from build123d import *

# Parameters (mm, degrees)
SKETCH_R        = 5
SKETCH_R_2      = 3.2
PAD_DEPTH       = 15
SKETCH002_R     = 6.1
POCKET001_DEPTH = 4
SKETCH003_R     = 11.1
POCKET_DEPTH    = 7.4


with BuildPart() as part:
    # Sketch → Pad (new body)
    with BuildSketch(Plane.XY):
        Polygon((20, 30), (20, 58), (62.3, 58), (62.3, 30), (82.3, 30), (82.3, 0), (0, 0), (0, 30), align=None)
        with Locations((41.15, 36.85)):
            Circle(SKETCH_R, mode=Mode.SUBTRACT)
        with Locations((11.15, 10)):
            Circle(SKETCH_R_2, mode=Mode.SUBTRACT)
        with Locations((31.15, 10)):
            Circle(SKETCH_R_2, mode=Mode.SUBTRACT)
        with Locations((51.15, 10)):
            Circle(SKETCH_R_2, mode=Mode.SUBTRACT)
        with Locations((71.15, 10)):
            Circle(SKETCH_R_2, mode=Mode.SUBTRACT)
    extrude(amount=PAD_DEPTH)

    # Sketch002 → Pocket001 (cut)
    with BuildSketch(Plane(origin=(0, 0, 0), x_dir=(1, 0, 0), z_dir=(0, 0, -1))):
        with Locations((11.15, -10)):
            Circle(SKETCH002_R)
        with Locations((31.15, -10)):
            Circle(SKETCH002_R)
        with Locations((51.15, -10)):
            Circle(SKETCH002_R)
        with Locations((71.15, -10)):
            Circle(SKETCH002_R)
    extrude(amount=-POCKET001_DEPTH, mode=Mode.SUBTRACT)

    # Sketch003 (on Face5 of Pocket001) → Pocket (cut)
    with BuildSketch(Plane.XY.offset(15)):
        with Locations((41.15, 36.85)):
            Circle(SKETCH003_R)
    extrude(amount=-POCKET_DEPTH, mode=Mode.SUBTRACT)


solid = part.part
Could you check a few things on this model? Use its own coordinates, in mm. A direction names the side the tool comes from. Give positions to 0.01 mm unless a question says otherwise; leave off trailing zeros. Order: outer loops, then holes, each group sorted by start corner. A loop starts at its lowest first (then second) coordinate and runs counter-clockwise, first axis right, second up. Notation, with made-up numbers: (25.25, 48) - (50.25, 48) arc R13 ccw to (50.25, 63) - close; hole circle Ø9 at (5, -28). An arc over 180 degrees is marked (long way). One line per item, written item: value. Start each with the question number.
1. Imagine slicing it at D-D on x = 10.5. List the corners of the cut face in (y, z) for me.
2. Imagine slicing it at B-B on z = 12.25. List the corners of the cut face in (x, y) for me.
3. Imagine slicing it at A-A on x = 41.15. List the corners of the cut face in (y, z) for me.
4. Imagine slicing it at C-C on y = 27. List the corners of the cut face in (x, z) for me, plus the area to 3 significant figures.
5. If I drill on probe 1 along X at (y, z) = (10, 12); probe 2 along X at (y, z) = (10, 1.4); probe 3 along X at (y, z) = (37, 12.5), over which ranges is the centre line in solid material (lowest first)?
6. Thinking about a two-plate mould opening in Y: for faces 5 (the face through (10, 30, 7)), 6 (the face through (9.828, 15.955, 1.972)), 7 (the face through (42, 29, 0)), which applies, +Y half, -Y half, draft (parallel to the pull), parting line (faces both ways), or undercut?
7. For faces 1 (the face through (46, 35, 7.6)), 2 (the face through (62.3, 44, 7)), 3 (the face through (20, 44, 7)), 4 (the face through (66.3, 13.7, 2)), which set-ups out of +Z, -Z, +X, -X, +Y, -Y let a thin tool reach every point of the face, with its end or its side?
8. For P1, Ø10, axis at x = 31.5, y = 9.5, coming from the -Z side; P2, Ø2, axis at x = 30.5, z = 6.5, coming from the -Y side; P3, Ø4.5, axis at y = 38, z = 4, coming from the +X side; P4, Ø20, axis at x = 41.15, y = 36.85, coming from the +Z side, each with a flat end and sliding along its axis, tell me the tip position at first contact or that it passes through.
Values:
1. outline: (0, 0) - (3.93, 0) - (3.93, 4) - (6.87, 4) - (6.87, 15) - (0, 15) - close; (13.13, 4) - (16.07, 4) - (16.07, 0) - (30, 0) - (30, 15) - (13.13, 15) - close
2. outline: (0, 0) - (82.3, 0) - (82.3, 30) - (62.3, 30) - (62.3, 58) - (20, 58) - (20, 30) - (0, 30) - close; hole circle Ø6.4 at (11.15, 10); hole circle Ø6.4 at (31.15, 10); hole circle Ø22.2 at (41.15, 36.85); hole circle Ø6.4 at (51.15, 10); hole circle Ø6.4 at (71.15, 10)
3. outline: (0, 0) - (31.85, 0) - (31.85, 7.6) - (25.75, 7.6) - (25.75, 15) - (0, 15) - close; (41.85, 0) - (58, 0) - (58, 15) - (47.95, 15) - (47.95, 7.6) - (41.85, 7.6) - close
4. outline: (0, 0) - (82.3, 0) - (82.3, 15) - (46.27, 15) - (46.27, 7.6) - (36.03, 7.6) - (36.03, 15) - (0, 15) - close
4. area: 1,160 mm²
5. probe 1: 0 to 7.95, 14.35 to 27.95, 34.35 to 47.95, 54.35 to 67.95, 74.35 to 82.3
5. probe 2: 0 to 5.05, 17.25 to 25.05, 37.25 to 45.05, 57.25 to 65.05, 77.25 to 82.3
5. probe 3: 20 to 30.05, 52.25 to 62.3
6. face 5: +Y half
6. face 6: undercut
6. face 7: draft
7. face 1: +Z
7. face 2: +Z, -Z, +X, +Y
7. face 3: +Z, -Z, -X, +Y
7. face 4: -Z
8. P1: z = 4
8. P2: y = 0
8. P3: x = 62.3
8. P4: z = 7.6
